```python
from build123d import *

# Parameters (mm, degrees)
F1_DEPTH = 25
F2_DEPTH = 5
F0_W     = 20
F0_H     = 6
F3_DEPTH = 10
F5_R     = 5
F7_D     = 5
F9_D     = 5


with BuildPart() as f1:
    # F0 (on Front) → F1 (new body, symmetric)
    with BuildSketch(Plane.XZ):
        Polygon((25, -7.5), (25, 7.5), (19, 7.5), (-25, 7.5), (-25, -7.5), align=None)
    extrude(amount=F1_DEPTH, both=True)

    # F0 (on Front) → F2 (join, symmetric)
    with BuildSketch(Plane.XZ):
        with BuildLine():
            Line((-25, 7.5), (19, 7.5))
            Line((19, 7.5), (19, 34.5))
            ThreePointArc((19, 34.5), (22.2218254069, 42.2781745931), (30, 45.5))
            add(Edge.make_bspline(
                [(-25, 7.5), (-11.6937831044, 29.0705016255), (6.4437664114, 45.5402298272), (30, 45.5)],
                knots=[0, 0, 0, 0, 66.8505796534, 66.8505796534, 66.8505796534, 66.8505796534], degree=3))
        make_face()
    extrude(amount=F2_DEPTH, both=True)

    # F0 (on Front) → F3 (join, symmetric)
    with BuildSketch(Plane.XZ):
        with BuildLine():
            Line((19, 7.5), (25, 7.5))
            Line((25, 7.5), (25, 34.5))
            ThreePointArc((25, 34.5), (26.4644660941, 38.0355339059), (30, 39.5))
            Line((30, 39.5), (65, 39.5))
            Line((65, 39.5), (65, 45.5))
            Line((65, 45.5), (30, 45.5))
            ThreePointArc((30, 45.5), (22.2218254069, 42.2781745931), (19, 34.5))
            Line((19, 34.5), (19, 7.5))
        make_face()
        with Locations((75, 42.5)):
            Rectangle(F0_W, F0_H)
    extrude(amount=F3_DEPTH, both=True)

    # F0 (on Front) → F4 (revolve)
    with BuildSketch(Plane.XZ):
        Polygon((85, 45.5), (85, 39.5), (85, 37.5), (105, 37.5), (105, 47.5), (85, 47.5), align=None)
    revolve(axis=Axis((85, 0, 42.5), (0, 0, 1)))

    # F5
    f5_edges = [f1.edges().sort_by_distance(p)[0] for p in [
        (25, 25, 0),
        (-25, 25, 0),
        (25, -25, 0),
        (-25, -25, 0),
    ]]
    fillet(f5_edges, radius=F5_R)

    # F7 (through all)
    with Locations(Plane.XY.offset(7.5)):
        with Locations((20, 20), (-20, 20), (20, -20), (-20, -20)):
            Hole(F7_D / 2)

    # F9 (through all)
    with Locations(Plane.XY.offset(47.5)):
        with Locations((85, 0), (73.5095148057, 11.4904851943), (96.4904851943, 11.4904851943), (73.5095148057, -11.4904851943), (96.8682619299, -11.0995354601), (85.1573778884, -16.249237896), (84.3727141619, 16.1917116493)):
            Hole(F9_D / 2)


solid = f1.part
```
Verification items for the finished model (mm, model axes). A direction names the side the tool comes from. Coordinates: 2 decimals unless noted, no trailing zeros. Order: outer loops, then holes, each group sorted by start corner. A loop starts at its lowest first (then second) coordinate and runs counter-clockwise, first axis right, second up. Notation, with made-up numbers: (-20.75, 61.5) - (2.25, 61.5) arc R18 cw to (2.25, 65.5) - close; hole circle Ø1 at (73, -19). An arc over 180 degrees is marked (long way). Return JSON: item names as keys, results as strings.
(1) Access from +Z, -Z, +X, -X, +Y, -Y to the whole of each face (thin tool, end or side, straight path). Record for faces 1 (the flat face through (25, 0, 9)), 2 (the cylindrical face through (26.43, -0.14, 38)), 3 (the flat face through (19, -8, 21)), 4 (the flat face through (2, 5, 23)).
Filled sheet:
{"face 1": "-Z, +X, +Y, -Y", "face 2": "-Z, +Y, -Y", "face 3": "+Z, -X, -Y", "face 4": "+Z, -X, +Y"}
(2) Go/stop test with flat-tipped pins: pin 1 (6.5 mm diameter, centred on x = 96.49, y = 11.49, fed in from +Z); pin 2 (22 mm diameter, centred on x = 40.5, y = 2.5, fed in from +Z); pin 3 (4 mm diameter, centred on y = -8.5, z = 10, fed in from -X); pin 4 (5 mm diameter, centred on x = 73.5, y = -9.5, fed in from -Z). Record where each tip stops, or that it passes through.
Filled sheet:
{"pin 1": "stops at z = 47.5", "pin 2": "stops at z = 45.5", "pin 3": "stops at x = 19", "pin 4": "stops at z = 37.5"}
(3) Section check A-A, the plane x = 85.5. Record the cut outline in (y, z).
Filled sheet:
{"outline": "(-19.99, 37.5) - (-18.73, 37.5) - (-18.73, 47.5) - (-19.99, 47.5) - close; (-13.77, 37.5) - (-2.45, 37.5) - (-2.45, 47.5) - (-13.77, 47.5) - close; (2.45, 37.5) - (13.96, 37.5) - (13.96, 47.5) - (2.45, 47.5) - close; (18.42, 37.5) - (19.99, 37.5) - (19.99, 47.5) - (18.42, 47.5) - close"}
(4) Section check B-B, the plane y = -7. Record the cut outline in (x, z) (3 decimals), and give its area (3 significant figures).
Filled sheet:
{"outline": "(-25, -7.5) - (25, -7.5) - (25, 34.5) arc R5 cw to (30, 39.5) - (66.265, 39.5) - (66.265, 37.5) - (103.735, 37.5) - (103.735, 47.5) - (66.265, 47.5) - (66.265, 45.5) - (30, 45.5) arc R11 ccw to (19, 34.5) - (19, 7.5) - (-25, 7.5) - close", "area": "1,580 mm^2"}
(5) Thickness scan on line 1 along Y through (x, z) = (-20, 2); line 2 along X through (y, z) = (-9, 14.5); line 3 along X through (y, z) = (1, 6). Record the ranges inside material, lowest first.
Filled sheet:
{"line 1": "y = -25 to -22.5, -17.5 to 17.5, 22.5 to 25", "line 2": "x = 19 to 25", "line 3": "x = -25 to 25"}
(6) Section check C-C, the plane z = 42.5. Give the number of separate pieces and of enclosed holes in the cut face, and give its area (3 significant figures).
Filled sheet:
{"separate pieces": "1", "enclosed holes": "7", "area": "2,080 mm^2"}
